```python
from build123d import *

# Parameters (mm, degrees)
SKETCH_1_R          = 1.5
EXTRUDE_1_DEPTH     = 11
CUT_EXTRUDE_START   = -9
CUT_EXTRUDE_1_DEPTH = 9
SKETCH_3_R          = 0.375
EXTRUDE_2_DEPTH     = 1.5


with BuildPart() as part:
    # Эскиз1 → Бобышка-Вытянуть1 (new body)
    with BuildSketch(Plane(origin=(0, 0, 0), x_dir=(1, 0, 0), z_dir=(0, 1, 0))):
        with Locations(Location((0, 0, 0), (0, 0, 270))):
            Circle(SKETCH_1_R)
    extrude(amount=EXTRUDE_1_DEPTH)

    # Эскиз2 → Вырез-Вытянуть1 (cut)
    with BuildSketch(Plane(origin=(0, 11, 0), x_dir=(1, 0, 0), z_dir=(0, 1, 0)).offset(CUT_EXTRUDE_START)):
        with BuildLine():
            Line((-0.9, -1.2), (-0.9, 1.2))
            ThreePointArc((-0.9, 1.2), (-1.5, 0), (-0.9, -1.2))
        make_face()
    extrude(amount=CUT_EXTRUDE_1_DEPTH, mode=Mode.SUBTRACT)

    # Эскиз3 → Бобышка-Вытянуть2 (add)
    with BuildSketch(Plane.XZ):
        with Locations(Location((0, 0, 0), (0, 0, 90))):
            Circle(SKETCH_3_R)
    extrude(amount=EXTRUDE_2_DEPTH)


solid = part.part
```
Check sheet for the modelled part. Datum: model origin and axes. Units: mm. A direction names the side the tool comes from. Give positions to 0.01 mm unless a question says otherwise; leave off trailing zeros. Write each loop counter-clockwise with the first axis right and the second up, starting at its lowest first coordinate (ties: lowest second). Pieces come first, ordered by that corner, then holes. Notation, with made-up numbers: (74, 73) - (122, 73) arc R33 ccw to (122, 102) - close; hole circle Ø11 at (-37, -6). An arc over 180 degrees is marked (long way). Answer as a JSON object with one key per item and string values. Group by question number.
1) Sectioned sample at B-B (z = -0.9). Record the cut outline in (x, y).
2) Sectioned sample at A-A (x = 0). Record the cut outline in (y, z) (3 decimals).
3) Sectioned sample at D-D (z = 0). Record the cut outline in (x, y) (3 decimals), then the cut area to 3 significant figures.
4) Sectioned sample at C-C (y = -0.5). Record the cut outline in (x, z) (3 decimals).
5) Access from +Z, -Z, +X, -X, +Y, -Y to the whole of each face (thin tool, end or side, straight path). Record for faces 1 (the face through (-0.9, 6, 0)), 2 (the face through (0, 11, 0)), 3 (the face through (0.4, 0, -0.4)).
6) Depth check by flat-ended pin: P1, Ø0.7, axis at x = -1, z = -0.5, coming from the +Y side; P2, Ø0.7, axis at y = 7.5, z = 0, coming from the -X side; P3, Ø1.5, axis at x = 1, z = 1, coming from the -Y side. Enter the tip coordinate at first touch or a pass-through.
7) Thickness scan on probe 1 along Y at (x, z) = (-0.1, 1.05); probe 2 along Z at (x, y) = (-0.1, 4.75). Record the ranges inside material, lowest first. Write a range as from..to.
Geometry results:
{
 "1": {"outline": "(-1.2, 0) - (1.2, 0) - (1.2, 11) - (-0.9, 11) - (-0.9, 2) - (-1.2, 2) - close"},
 "2": {"outline": "(-1.5, -0.375) - (0, -0.375) - (0, -1.5) - (11, -1.5) - (11, 1.5) - (0, 1.5) - (0, 0.375) - (-1.5, 0.375) - close"},
 "3": {"outline": "(-1.5, 0) - (-0.375, 0) - (-0.375, -1.5) - (0.375, -1.5) - (0.375, 0) - (1.5, 0) - (1.5, 11) - (-0.9, 11) - (-0.9, 2) - (-1.5, 2) - close", "area": "28.7 mm^2"},
 "4": {"outline": "circle Ø0.75 at (0, 0)"},
 "5": {"face 1": "+Z, -Z, -X, +Y", "face 2": "+Z, -Z, +X, -X, +Y", "face 3": "-Y"},
 "6": {"P1": "stops at y = 11", "P2": "stops at x = -0.9", "P3": "stops at y = 0"},
 "7": {"probe 1": "y = 0..11", "probe 2": "z = -1.5..1.5"}
}
